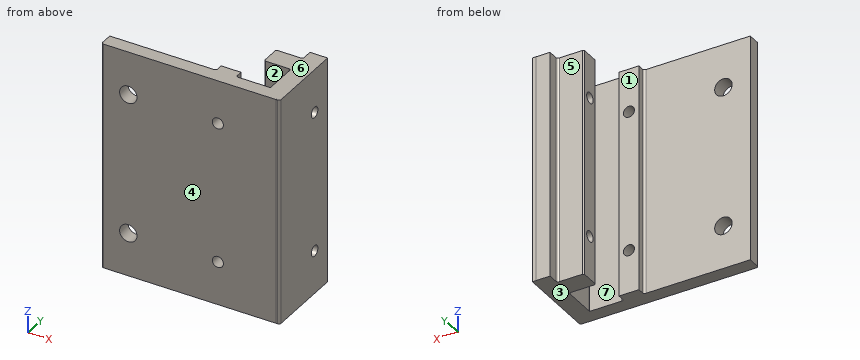
from build123d import *

# Parameters (mm, degrees)
BOSS_EXTRUDE1_DEPTH        = 66.675
CUT_EXTRUDE1_REACH         = 75.8
CUT_EXTRUDE2_REACH         = 75.8
SKETCH6_W                  = 66.675
SKETCH6_H                  = 4.064
BOSS_EXTRUDE2_DEPTH        = 22.21738
F_10_CLEARANCE_HOLE1_D     = 5.1054
SKETCH12_W                 = 5.842
SKETCH12_H                 = 5.49275
CUT_EXTRUDE4_DEPTH         = 77.796738301
F_4_CLEARANCE_HOLE1_D      = 3.2639
SKETCH19_W                 = 66.675
SKETCH19_H                 = 23.410344024
BOSS_EXTRUDE7_DEPTH        = 1.12776
F_1_8_0_1250_DOWEL_HOLE1_D = 3.175
SKETCH20_W                 = 1.016
SKETCH20_H                 = 4.064
CUT_EXTRUDE5_DEPTH         = 77.796821417
FILLET1_R                  = 0.635


with BuildPart() as part:
    # Sketch1 → Boss-Extrude1 (new body)
    with BuildSketch(Plane(origin=(0, 0, -3683), x_dir=(-1, 0, 0), z_dir=(0, 0, -1))):
        with BuildLine():
            Line((7.945265893, 3.588862728), (-1.198734107, 3.588862728))
            ThreePointArc((-1.198734107, 3.588862728), (-1.647746913, 3.774849922), (-1.833734107, 4.223862728))
            Line((-1.833734107, 4.223862728), (-1.833734107, 5.747862728))
            ThreePointArc((-1.833734107, 5.747862728), (-1.647746913, 6.196875535), (-1.198734107, 6.382862728))
            Line((-1.198734107, 6.382862728), (1.621629442, 6.382862728))
            Line((1.621629442, 6.382862728), (1.621629442, 6.890862686))
            Line((1.621629442, 6.890862686), (-2.214734107, 11.462862728))
            Line((-2.214734107, 11.462862728), (-7.294734107, 11.462862728))
            Line((-7.294734107, 11.462862728), (-11.131097656, 6.890862686))
            Line((-11.131097656, 6.890862686), (-11.131097656, 6.382862728))
            Line((-11.131097656, 6.382862728), (-8.310734107, 6.382862728))
            ThreePointArc((-8.310734107, 6.382862728), (-7.861721301, 6.196875535), (-7.675734107, 5.747862728))
            Line((-7.675734107, 5.747862728), (-7.675734107, 4.223862728))
            ThreePointArc((-7.675734107, 4.223862728), (-7.861721301, 3.774849922), (-8.310734107, 3.588862728))
            Line((-8.310734107, 3.588862728), (-17.454734107, 3.588862728))
            Line((-17.454734107, 3.588862728), (-17.727921752, 3.588862728))
            Line((-17.727921752, 3.588862728), (-17.727921752, 3.858842754))
            Line((-17.727921752, 3.858842754), (-17.728361466, 13.002372481))
            ThreePointArc((-17.728361466, 13.002372481), (-17.542256287, 13.451715967), (-17.092921752, 13.637842754))
            Line((-17.092921752, 13.637842754), (-15.568921752, 13.637842754))
            ThreePointArc((-15.568921752, 13.637842754), (-15.119908946, 13.45185556), (-14.933921752, 13.002842754))
            Line((-14.933921752, 13.002842754), (-14.933921752, 10.182479205))
            Line((-14.933921752, 10.182479205), (-14.425921794, 10.182479205))
            Line((-14.425921794, 10.182479205), (-9.853921752, 14.018842754))
            Line((-9.853921752, 14.018842754), (-9.853921752, 19.098842754))
            Line((-9.853921752, 19.098842754), (-14.425921794, 22.935206303))
            Line((-14.425921794, 22.935206303), (-14.933921752, 22.935206303))
            Line((-14.933921752, 22.935206303), (-14.933921752, 20.114842754))
            ThreePointArc((-14.933921752, 20.114842754), (-15.119908946, 19.665829948), (-15.568921752, 19.479842754))
            Line((-15.568921752, 19.479842754), (-17.092921752, 19.479842754))
            ThreePointArc((-17.092921752, 19.479842754), (-17.542476558, 19.66604812), (-17.728703542, 20.11559397))
            Line((-17.728703542, 20.11559397), (-17.728839138, 22.935206303))
            Line((-17.728839138, 22.935206303), (-21.787214199, 22.935206303))
            Line((-21.787214199, 22.935206303), (-21.791921752, 3.859128788))
            Line((-21.791921752, 3.859128788), (-21.791921752, 3.588862728))
            Line((-21.791921752, 3.588862728), (-21.791921752, -0.475137272))
            Line((-21.791921752, -0.475137272), (-17.727921752, -0.475137272))
            Line((-17.727921752, -0.475137272), (-17.454774021, -0.475137272))
            Line((-17.454774021, -0.475137272), (7.945225979, -0.475137272))
            Line((7.945225979, -0.475137272), (8.215492039, -0.475137272))
            Line((8.215492039, -0.475137272), (8.215492039, 3.588862728))
            Line((8.215492039, 3.588862728), (7.945265893, 3.588862728))
        make_face()
    extrude(amount=BOSS_EXTRUDE1_DEPTH)

    # Sketch2 → Cut-Extrude1 (cut, up to next)
    with BuildSketch(Plane.XY.offset(-3683), mode=Mode.PRIVATE) as cut_extrude1_sk1:
        with BuildLine():
            Line((11.131097656, 6.890862686), (11.131097656, 6.382862728))
            Line((11.131097656, 6.382862728), (8.310734107, 6.382862728))
            ThreePointArc((8.310734107, 6.382862728), (7.861721301, 6.196875535), (7.675734107, 5.747862728))
            Line((7.675734107, 5.747862728), (7.675734107, 11.00880461))
            Line((7.675734107, 11.00880461), (11.131097656, 6.890862686))
        make_face()
    cut_extrude1_tool1 = extrude(cut_extrude1_sk1.sketch, amount=-CUT_EXTRUDE1_REACH, mode=Mode.PRIVATE) & part.part
    # Sketch2 → Cut-Extrude1 (cut, up to next)
    with BuildSketch(Plane.XY.offset(-3683), mode=Mode.PRIVATE) as cut_extrude1_sk2:
        with BuildLine():
            Line((1.833734107, 5.747862728), (1.833734107, 11.00880461))
            Line((1.833734107, 11.00880461), (-1.621629442, 6.890862686))
            Line((-1.621629442, 6.890862686), (-1.621629442, 6.382862728))
            Line((-1.621629442, 6.382862728), (1.198734107, 6.382862728))
            ThreePointArc((1.198734107, 6.382862728), (1.647746913, 6.196875535), (1.833734107, 5.747862728))
        make_face()
    cut_extrude1_tool2 = extrude(cut_extrude1_sk2.sketch, amount=-CUT_EXTRUDE1_REACH, mode=Mode.PRIVATE) & part.part
    add(cut_extrude1_tool1.solids().sort_by_distance((8.930632, 7.925168, -3683))[0], mode=Mode.SUBTRACT)
    add(cut_extrude1_tool2.solids().sort_by_distance((0.578837, 7.925168, -3683))[0], mode=Mode.SUBTRACT)

    # Sketch3 → Cut-Extrude2 (cut, up to next)
    with BuildSketch(Plane.XY.offset(-3683), mode=Mode.PRIVATE) as cut_extrude2_sk1:
        with BuildLine():
            Line((15.568921752, 19.479842754), (10.307979871, 19.479842754))
            Line((10.307979871, 19.479842754), (14.425921794, 22.935206303))
            Line((14.425921794, 22.935206303), (14.933921752, 22.935206303))
            Line((14.933921752, 22.935206303), (14.933921752, 20.114842754))
            ThreePointArc((14.933921752, 20.114842754), (15.119908946, 19.665829948), (15.568921752, 19.479842754))
        make_face()
    cut_extrude2_tool1 = extrude(cut_extrude2_sk1.sketch, amount=-CUT_EXTRUDE2_REACH, mode=Mode.PRIVATE) & part.part
    # Sketch3 → Cut-Extrude2 (cut, up to next)
    with BuildSketch(Plane.XY.offset(-3683), mode=Mode.PRIVATE) as cut_extrude2_sk2:
        with BuildLine():
            Line((10.307979871, 13.637842754), (14.425921794, 10.182479205))
            Line((14.425921794, 10.182479205), (14.933921752, 10.182479205))
            Line((14.933921752, 10.182479205), (14.933921752, 13.002842754))
            ThreePointArc((14.933921752, 13.002842754), (15.119908946, 13.45185556), (15.568921752, 13.637842754))
            Line((15.568921752, 13.637842754), (10.307979871, 13.637842754))
        make_face()
    cut_extrude2_tool2 = extrude(cut_extrude2_sk2.sketch, amount=-CUT_EXTRUDE2_REACH, mode=Mode.PRIVATE) & part.part
    add(cut_extrude2_tool1.solids().sort_by_distance((13.391616, 20.73474, -3683))[0], mode=Mode.SUBTRACT)
    add(cut_extrude2_tool2.solids().sort_by_distance((13.391616, 12.382945, -3683))[0], mode=Mode.SUBTRACT)

    # Sketch6 → Boss-Extrude2 (add)
    with BuildSketch(Plane.ZY.offset(8.215492039)):
        with Locations((-3716.3375, 1.556862728)):
            Rectangle(SKETCH6_W, SKETCH6_H)
    extrude(amount=BOSS_EXTRUDE2_DEPTH)

    # #10 Clearance Hole1 (through all)
    with Locations(Plane(origin=(0, 3.588862728, 0), x_dir=(1, 0, 0), z_dir=(0, 1, 0))):
        with Locations((-21.530172039, 3736.975), (-21.530172039, 3695.7)):
            Hole(F_10_CLEARANCE_HOLE1_D / 2)

    # Sketch12 → Cut-Extrude4 (cut, through all)
    with BuildSketch(Plane(origin=(0, 0, -3749.675), x_dir=(-1, 0, 0), z_dir=(0, 0, -1))):
        with Locations((-4.754734107, 8.716487728)):
            Rectangle(SKETCH12_W, SKETCH12_H)
    extrude(amount=-CUT_EXTRUDE4_DEPTH, mode=Mode.SUBTRACT)

    # #4 Clearance Hole1 (through all)
    with Locations(Plane(origin=(0, 5.970112728, 0), x_dir=(1, 0, 0), z_dir=(0, 1, 0))):
        with Locations((4.754734107, 3736.975), (4.754734107, 3695.7)):
            Hole(F_4_CLEARANCE_HOLE1_D / 2)

    # Sketch19 → Boss-Extrude7 (add)
    with BuildSketch(Plane(origin=(21.792872772, 0.005377998, 0), x_dir=(0, 0, -1), z_dir=(0.9999999695503556, 0.0002467778108309542, 0))):
        with Locations((3716.3375, 11.224656992)):
            Rectangle(SKETCH19_W, SKETCH19_H)
    extrude(amount=BOSS_EXTRUDE7_DEPTH)

    # 1/8 (0.1250) Dowel Hole1 (through all)
    with Locations(Plane.ZY.offset(-9.853921752)):
        with Locations((-3736.975, 16.558842754), (-3695.7, 16.558842754)):
            Hole(F_1_8_0_1250_DOWEL_HOLE1_D / 2)

    # Sketch20 → Cut-Extrude5 (cut, through all)
    with BuildSketch(Plane.XY.offset(-3683)):
        with Locations((-29.924872039, 1.556862728)):
            Rectangle(SKETCH20_W, SKETCH20_H)
    extrude(amount=-CUT_EXTRUDE5_DEPTH, mode=Mode.SUBTRACT)

    # Fillet1
    fillet1_edges = [part.edges().sort_by_distance(p)[0] for p in [
        (22.920751318, -0.474858701, -3716.3375),
        (-29.416872039, -0.475137272, -3716.3375),
    ]]
    fillet(fillet1_edges, radius=FILLET1_R)


solid = part.part
The model under review builds one solid part; all positions refer to its coordinate system, in mm. Face numbers are marked on the shaded views. A direction names the side the tool comes from. Round coordinates to 2 decimals unless told otherwise and drop trailing zeros. Loops run counter-clockwise (first coordinate to the right, second up) from the corner with the lowest first, then second, coordinate; pieces in that order, holes last. Notation, with made-up numbers: (72, 80.5) -> (131, 80.5) arc R13 ccw to (131, 104.5) -> close; hole circle Ø6 at (58, 40.5). An arc over 180 degrees is marked (long way). Write item = value, one per line. Start each with the question number.
Item 1: To check wall thickness, follow L1, parallel to X at y = 5.75, z = -3734.5; L2, parallel to Y at x = 17, z = -3707; L3, parallel to X at y = 4.75, z = -3695.7. State the ranges of each line that lie inside material, in increasing order.
Item 2: Take a section at A-A on x = 12. Give the boundary of the cut face in (y, z) (1 decimal), plus the area to 3 significant figures.
Item 3: Take a section at B-B on z = -3720. Give the boundary of the cut face in (x, y) (3 decimals).
Item 4: Insertion check: pin 1 (4.5 mm diameter, centred on x = 11.5, z = -3707, fed in from +Y); pin 2 (10 mm diameter, centred on x = -10.5, z = -3698.5, fed in from +Y); pin 3 (3 mm diameter, centred on y = 16.56, z = -3736.98, fed in from +X); pin 4 (3 mm diameter, centred on x = 4.5, z = -3713, fed in from +Y). Each pin has a flat end and moves straight along its axis. Give the tip position at first contact, or say it passes through.
Item 5: Mouldability with a two-part tool opening along Y and no side actions: class the marked faces 4, 5, 6 and 7 as released by +Y, released by -Y, zero draft, split by the parting line, or undercut.
Item 6: Take a section at D-D on y = 21. Give the boundary of the cut face in (x, z) (3 decimals).
Item 7: For the marked faces 1, 2 and 3, list the 3-axis set-ups (+Z, -Z, +X, -X, +Y, -Y) from which the entire face can be reached by the end or side of a thin tool; tool diameter is ignored.
Item 8: Take a section at C-C on x = -6. Give the boundary of the cut face in (y, z) (3 decimals), plus the area to 3 significant figures.
Result:
q1.L1 = 1.83 to 7.68, 17.73 to 22.92
q1.L2 = -0.48 to 3.59, 13.64 to 19.48
q1.L3 = 1.83 to 3.12, 6.39 to 7.68, 17.73 to 22.92
q2.outline = (-0.5, -3749.7) -> (3.6, -3749.7) -> (3.6, -3683) -> (-0.5, -3683) -> close; (13.6, -3749.7) -> (19.5, -3749.7) -> (19.5, -3683) -> (13.6, -3683) -> close; hole circle Ø3.2 at (16.6, -3737); hole circle Ø3.2 at (16.6, -3695.7)
q2.area = 645 mm²
q3.outline = (-29.417, 0.16) arc R0.635 ccw to (-28.782, -0.475) -> (21.792, -0.475) -> (21.792, 3.859) -> (21.793, -0.475) -> (22.286, -0.475) arc R0.635 ccw to (22.921, 0.16) -> (22.915, 22.935) -> (21.787, 22.935) -> (17.729, 22.935) -> (17.729, 20.116) arc R0.636 cw to (17.093, 19.48) -> (10.308, 19.48) -> (9.854, 19.099) -> (9.854, 14.019) -> (10.308, 13.638) -> (17.093, 13.638) arc R0.635 cw to (17.728, 13.002) -> (17.728, 3.859) -> (17.728, 3.589) -> (8.311, 3.589) arc R0.635 cw to (7.676, 4.224) -> (7.676, 5.97) -> (1.834, 5.97) -> (1.834, 4.224) arc R0.635 cw to (1.199, 3.589) -> (-29.417, 3.589) -> close
q4.pin_1 = 19.48
q4.pin_2 = 3.59
q4.pin_3 = through
q4.pin_4 = 5.97
q5.face_4 = released by -Y
q5.face_5 = released by +Y
q5.face_6 = zero draft
q5.face_7 = undercut
q6.outline = (17.729, -3749.675) -> (22.915, -3749.675) -> (22.915, -3683) -> (17.729, -3683) -> close
q7.face_1 = +Z, -Z, -X, +Y
q7.face_2 = +Z, -Z, -X
q7.face_3 = -Z, +X, -X, +Y, -Y
q8.outline = (-0.475, -3749.675) -> (3.589, -3749.675) -> (3.589, -3683) -> (-0.475, -3683) -> close
q8.area = 271 mm²
